from build123d import *

# Parameters (mm, degrees)
F1_DEPTH = 25
F2_DEPTH = 10
F3_R     = 5
F5_DEPTH = 3


with BuildPart() as f1:
    # F0 (on Front) → F1 (new body)
    with BuildSketch(Plane.XZ):
        with BuildLine():
            ThreePointArc((17.495668, -0.389351), (16.123041, 2.842927), (16.307385, 6.349741))
            ThreePointArc((16.307385, 6.349741), (15.155445, 8.75), (13.652729, 10.947739))
            ThreePointArc((13.652729, 10.947739), (10.523567, 12.541499), (8.410647, 15.346368))
            ThreePointArc((8.410647, 15.346368), (5.985353, 16.444621), (3.421526, 17.16226))
            ThreePointArc((3.421526, 17.16226), (0, 16.371764), (-3.421526, 17.16226))
            ThreePointArc((-3.421526, 17.16226), (-5.985353, 16.444621), (-8.410647, 15.346368))
            ThreePointArc((-8.410647, 15.346368), (-10.523567, 12.541499), (-13.652729, 10.947739))
            ThreePointArc((-13.652729, 10.947739), (-15.155445, 8.75), (-16.307385, 6.349741))
            ThreePointArc((-16.307385, 6.349741), (-16.123041, 2.842927), (-17.495668, -0.389351))
            ThreePointArc((-17.495668, -0.389351), (-17.234136, -3.038843), (-16.573716, -5.618001))
            ThreePointArc((-16.573716, -5.618001), (-14.178364, -8.185882), (-13.15219, -11.544259))
            ThreePointArc((-13.15219, -11.544259), (-11.248783, -13.405778), (-9.085022, -14.957018))
            ThreePointArc((-9.085022, -14.957018), (-5.599473, -15.384426), (-2.654655, -17.29748))
            ThreePointArc((-2.654655, -17.29748), (0, -17.5), (2.654655, -17.29748))
            ThreePointArc((2.654655, -17.29748), (5.599473, -15.384426), (9.085022, -14.957018))
            ThreePointArc((9.085022, -14.957018), (11.248783, -13.405778), (13.15219, -11.544259))
            ThreePointArc((13.15219, -11.544259), (14.178364, -8.185882), (16.573716, -5.618001))
            ThreePointArc((16.573716, -5.618001), (17.234136, -3.038843), (17.495668, -0.389351))
        make_face()
        with BuildLine():
            ThreePointArc((3, 4), (4.472136, 2.236068), (5, 0))
            ThreePointArc((5, 0), (-2.236068, -4.472136), (-3, 4))
            ThreePointArc((-3, 4), (0, 5), (3, 4))
        make_face(mode=Mode.SUBTRACT)
        with BuildLine():
            Line((-3, 4), (3, 4))
            ThreePointArc((3, 4), (0, 5), (-3, 4))
        make_face()
        with BuildLine():
            ThreePointArc((-3, 4), (-2.236068, -4.472136), (5, 0))
            ThreePointArc((5, 0), (4.472136, 2.236068), (3, 4))
            Line((3, 4), (-3, 4))
        make_face()
    extrude(amount=F1_DEPTH)

    # F0 (on Front) → F2 (cut)
    with BuildSketch(Plane.XZ):
        with BuildLine():
            ThreePointArc((-3, 4), (-2.236068, -4.472136), (5, 0))
            ThreePointArc((5, 0), (4.472136, 2.236068), (3, 4))
            Line((3, 4), (-3, 4))
        make_face()
    extrude(amount=F2_DEPTH, mode=Mode.SUBTRACT)

    # F3
    f3_edges = [f1.edges().sort_by_distance(p)[0] for p in [
        (-5.599473, -25, -15.384426),
        (0, -25, -17.5),
        (5.599473, -25, -15.384426),
        (11.248783, -25, -13.405778),
        (14.178364, -25, -8.185882),
        (17.234136, -25, -3.038843),
        (16.123041, -25, 2.842927),
        (15.155445, -25, 8.75),
        (10.523567, -25, 12.541499),
        (5.985353, -25, 16.444621),
        (0, -25, 16.371764),
        (-5.985353, -25, 16.444621),
        (-10.523567, -25, 12.541499),
        (-15.155445, -25, 8.75),
        (-16.123041, -25, 2.842927),
        (-17.234136, -25, -3.038843),
        (-14.178364, -25, -8.185882),
        (-11.248783, -25, -13.405778),
    ]]
    fillet(f3_edges, radius=F3_R)

    # F4 (on face) → F5 (cut)
    with BuildSketch(Plane.XZ.offset(25)):
        Polygon((3.03, 0), (0, 9.24), (0, 0), align=None)
        Polygon((0, 0), (0, 9.24), (-3.03, 0), align=None)
    extrude(amount=-F5_DEPTH, mode=Mode.SUBTRACT)


solid = f1.part
Geometry check sheet. Reference: the model listing, model coordinates, mm. A direction names the side the tool comes from. Round coordinates to 2 decimals unless told otherwise and drop trailing zeros. Write each loop counter-clockwise with the first axis right and the second up, starting at its lowest first coordinate (ties: lowest second). Pieces come first, ordered by that corner, then holes.
Item 1: Section check B-B (y = -8.5). Record the boundary of the cut face in (x, z).
Determined:
outline: (-17.5, -0.39) arc R17.5 ccw to (-16.57, -5.62) arc R7.8 cw to (-13.15, -11.54) arc R17.5 ccw to (-9.09, -14.96) arc R7.8 cw to (-2.65, -17.3) arc R17.5 ccw to (2.65, -17.3) arc R7.8 cw to (9.09, -14.96) arc R17.5 ccw to (13.15, -11.54) arc R7.8 cw to (16.57, -5.62) arc R17.5 ccw to (17.5, -0.39) arc R7.8 cw to (16.31, 6.35) arc R17.5 ccw to (13.65, 10.95) arc R7.8 cw to (8.41, 15.35) arc R17.5 ccw to (3.42, 17.16) arc R7.8 cw to (-3.42, 17.16) arc R17.5 ccw to (-8.41, 15.35) arc R7.8 cw to (-13.65, 10.95) arc R17.5 ccw to (-16.31, 6.35) arc R7.8 cw to start; hole (-3, 4) arc R5 ccw (long way) to (3, 4) - close
Item 2: Access from +Z, -Z, +X, -X, +Y, -Y to the whole of each face (thin tool, end or side, straight path). Record for faces 1 (the face through (-1.494, -23.521, 4.685)), 2 (the face through (-5.646, -9.86, -15.368)), 3 (the face through (0, -10, 0)).
Determined:
face 1: -Y
face 2: -Z, +Y, -Y
face 3: +Y
Item 3: Material ranges on line 1 along Z through (x, y) = (0, -8); line 2 along Z through (x, y) = (1, -7.25); line 3 along X through (y, z) = (-2, -3), recorded low to high.
Determined:
line 1: z = -17.5 to -5, 4 to 16.37
line 2: z = -17.47 to -4.9, 4 to 16.44
line 3: x = -17.24 to -4, 4 to 17.24
Item 4: Mould release check, pull along X, two halves, no side actions. Record for faces 4 (the face through (-5.95, -9.86, 16.457)), 5 (the face through (5.553, -9.86, -15.402)), 6 (the face through (1.536, -23.521, 4.555)), 7 (the face through (4, 0, 4)): +X half, -X half, draft (parallel to the pull), parting line (faces both ways), or undercut.
Determined:
face 4: -X half
face 5: undercut
face 6: undercut
face 7: draft
Item 5: Section check A-A (y = -12). Record the boundary of the cut face in (x, z).
Determined:
outline: (-17.5, -0.39) arc R17.5 ccw to (-16.57, -5.62) arc R7.8 cw to (-13.15, -11.54) arc R17.5 ccw to (-9.09, -14.96) arc R7.8 cw to (-2.65, -17.3) arc R17.5 ccw to (2.65, -17.3) arc R7.8 cw to (9.09, -14.96) arc R17.5 ccw to (13.15, -11.54) arc R7.8 cw to (16.57, -5.62) arc R17.5 ccw to (17.5, -0.39) arc R7.8 cw to (16.31, 6.35) arc R17.5 ccw to (13.65, 10.95) arc R7.8 cw to (8.41, 15.35) arc R17.5 ccw to (3.42, 17.16) arc R7.8 cw to (-3.42, 17.16) arc R17.5 ccw to (-8.41, 15.35) arc R7.8 cw to (-13.65, 10.95) arc R17.5 ccw to (-16.31, 6.35) arc R7.8 cw to start
Item 6: Go/stop test with flat-tipped pins: pin 1 Ø3 at (x, y) = (8.5, -4.5) entering from +Z; pin 2 Ø4 at (y, z) = (-5, -4) entering from -X; pin 3 Ø1.5 at (x, y) = (0.5, -23.5) entering from +Z. Record where each tip stops, or that it passes through.
Determined:
pin 1: stops at z = 16.04
pin 2: stops at x = -17.39
pin 3: stops at z = 15.56
